The model under review builds one solid part; all positions refer to its coordinate system, in mm. Face numbers are marked on the shaded views. Give positions to 0.01 mm unless a question says otherwise; leave off trailing zeros. Return JSON: item names as keys, results as strings.
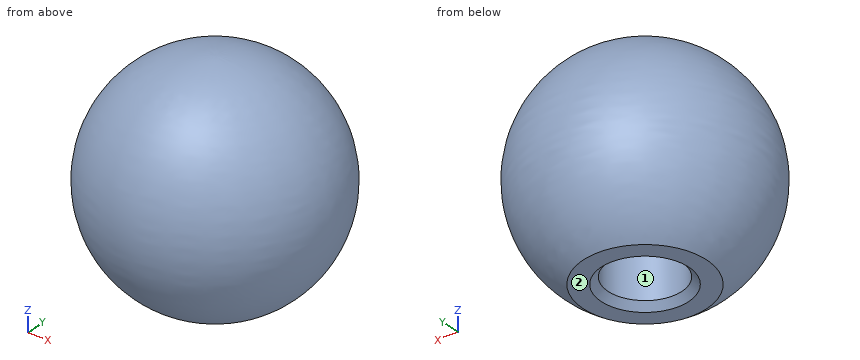
Autodesk Inventor part; units mm, degrees
ref_plane "YZ Plane" through (0, 0, 0) normal (1, 0, 0) x (0, 1, 0)
ref_plane "XZ Plane" through (0, 0, 0) normal (0, 1, 0) x (-1, 0, 0)
ref_plane "XY Plane" through (0, 0, 0) normal (0, 0, 1) x (1, 0, 0)
sketch "Sketch5" plane through (0, 0, 0) normal (0, 1, 0) x (-1, 0, 0)
  arc A0 (0, 5) -> (-2.7129, -4.2) centre (0, 0) ccw
  line L0 (-2.7129, -4.2) -> (0, -4.2)
  line L1 (0, 5) -> (0, -4.2)
  dimension "d15" = 10
  dimension "d16" = 9.2
revolve "Revolution1" add sketch "Sketch5" angle 360 about axis through (0, 0, 5) along (0, 0, -1)
sketch "Sketch6" plane through (0, 0, -4.2) normal (0, 0, -1) x (-1, 0, 0)
  circle A0 centre (0, 0) radius 2.7129
hole "Hole1" at (0, 0, -4.2) direction (0, 0, 1) diameter 3.242 depth 7 tip angle 118
chamfer "Chamfer1" distance 0.3 angle 45 1 edges at (0, -1.621, -4.2)
properties part number "m3 6" material "Steel"
1) Insertion check: pin 1 (1.5 mm diameter, centred on x = 0, z = 1, fed in from -Y); pin 2 (2 mm diameter, centred on x = -2, y = -1.5, fed in from +Z); pin 3 (2 mm diameter, centred on x = 2, z = 3, fed in from -Y). Each pin has a flat end and moves straight along its axis. Give the tip position at first contact, or say it passes through.
From the geometry:
{"pin 1": "y = -4.99", "pin 2": "z = 4.77", "pin 3": "y = -4.27"}
2) Wall thickness on L1, parallel to X at y = 0, z = 0; L2, parallel to X at y = 0, z = 1.5; L3, parallel to Y at x = 0.5, z = 1: over which ranges is each line inside the solid? List them lowest first. Write a range as from..to.
From the geometry:
{"L1": "-5..-1.62, 1.62..5", "L2": "-4.77..-1.62, 1.62..4.77", "L3": "-4.87..-1.54, 1.54..4.87"}
3) The part is to be moulded in two halves that separate along X. For the marked faces 1 and 2, say which applies: released by +X, released by -X, zero draft, split by the parting line, or undercut.
From the geometry:
{"face 1": "undercut", "face 2": "zero draft"}
